Design review of the part built by this model. Coordinates are the model's own, in mm. Coordinates: 2 decimals unless noted, no trailing zeros. Write each loop counter-clockwise with the first axis right and the second up, starting at its lowest first coordinate (ties: lowest second). Pieces come first, ordered by that corner, then holes.
Q1. To check wall thickness, follow probe 1 along Y at (x, z) = (19, -5); probe 2 along Y at (x, z) = (-15, -7.25); probe 3 along X at (y, z) = (228.5, -3). State the ranges of each line that lie inside material, in increasing order.
Q2. Add section C-C, the plane y = 156. Give the boundary of the cut face in (x, z).
Q3. The part is to be moulded in two halves that separate along X. For faces 1 (the face through (-165, -153.2, -4.9)), 2 (the face through (-0.286, 264.503, -4.93)), 3 (the face through (165, 153.2, -4.9)), say which applies: +X half, -X half, draft (parallel to the pull), parting line (faces both ways), or undercut.
Q4. Add section A-A, the plane z = -6.75. Give the number of separate pieces and of enclosed holes in the cut face, plus the area to 3 significant figures.
Q5. Clearance check with flat-ended pins moving along their axes: pin 1 Ø2.5 at (x, y) = (-281.7, 8) entering from +Z; pin 2 Ø5 at (y, z) = (284, -4.5) entering from -X; pin 3 Ø5 at (x, z) = (41, -4) entering from +Y; pin 4 Ø1.5 at (y, z) = (-81, -1.5) entering from +X. State where each tip first meets the part, or that it passes through.
Q6. Add section B-B, the plane x = 0. Give the boundary of the cut face in (y, z), plus the area to 3 significant figures.
Autodesk Inventor part; units mm, degrees
ref_plane "YZ Plane" through (0, 0, 0) normal (1, 0, 0) x (0, 1, 0)
ref_plane "XZ Plane" through (0, 0, 0) normal (0, 1, 0) x (-1, 0, 0)
ref_plane "XY Plane" through (0, 0, 0) normal (0, 0, 1) x (1, 0, 0)
sketch "Sketch2" plane through (0, 0, 0) normal (0, 0, 1) x (1, 0, 0)
  circle A0 centre (0, 277.5) radius 8 construction
  circle A1 centre (0, 277.5) radius 13
  circle A2 centre (0, 277.5) radius 10.5 construction
  line L0 (25, 287.5) -> (-25, 287.5) construction
  line L1 (-25, 287.5) -> (-25, 222.5) construction
  line L2 (-25, 222.5) -> (25, 222.5) construction
  line L3 (25, 222.5) -> (25, 287.5) construction
  circle A3 centre (15, 228.5) radius 2.7
  circle A4 centre (-15, 228.5) radius 2.7
  circle A5 centre (-19, 277.5) radius 2.7
  circle A6 centre (19, 277.5) radius 2.7
  circle A7 centre (0, -277.5) radius 8 construction
  circle A8 centre (0, -277.5) radius 13
  circle A9 centre (0, -277.5) radius 10.5 construction
  line L4 (25, -287.5) -> (-25, -287.5) construction
  line L5 (-25, -287.5) -> (-25, -222.5) construction
  line L6 (-25, -222.5) -> (25, -222.5) construction
  line L7 (25, -222.5) -> (25, -287.5) construction
  circle A10 centre (-15, -228.5) radius 2.7
  circle A11 centre (15, -228.5) radius 2.7
  circle A12 centre (-19, -277.5) radius 2.7
  circle A13 centre (19, -277.5) radius 2.7
  line L8 (10.5, -277.5) -> (10.5, -287.5) construction
  line L9 (-10.5, -277.5) -> (-10.5, -287.5) construction
  line L10 (10.5, 277.5) -> (10.5, 287.5) construction
  line L11 (-10.5, 277.5) -> (-10.5, 287.5) construction
  circle A14 centre (281.7, 0) radius 5.25
  circle A15 centre (289.7, 0) radius 1.6
  circle A16 centre (281.7, 8) radius 1.6
  circle A17 centre (273.7, 0) radius 1.6
  circle A18 centre (281.7, -8) radius 1.6
  circle A19 centre (-281.7, 0) radius 5.25
  circle A20 centre (-289.7, 0) radius 1.6
  circle A21 centre (-281.7, -8) radius 1.6
  circle A22 centre (-273.7, 0) radius 1.6
  circle A23 centre (-281.7, 8) radius 1.6
  line L12 (0, -318.1981) -> (318.1981, 0)
  line L13 (318.1981, 0) -> (0, 318.1981)
  line L14 (0, 318.1981) -> (-318.1981, 0)
  line L15 (-318.1981, 0) -> (0, -318.1981)
  line L16 (0, -318.1981) -> (0, 318.1981) construction
  line L17 (318.1981, 0) -> (-318.1981, 0) construction
  line L18 (0, -318.1981) -> (450, -318.1981) construction
  line L19 (300.5, 17.6981) -> (300.5, -17.6981)
  line L20 (-300.5, 17.6981) -> (-300.5, -17.6981)
  line L21 (-20.6981, 297.5) -> (20.6981, 297.5) construction
  line L22 (-25.6981, 292.5) -> (25.6981, 292.5)
  line L23 (-20.6981, -297.5) -> (20.6981, -297.5) construction
  line L24 (-25.6981, -292.5) -> (25.6981, -292.5)
  line L25 (-9.5, 297.5) -> (-3.976, 284.442) construction
  line L26 (9.5, 297.5) -> (3.976, 284.442) construction
  line L27 (-14.929, 297.5) -> (-9.9883, 285.8207)
  line L28 (14.929, 297.5) -> (9.9883, 285.8207)
  line L29 (-9.5, -297.5) -> (-3.976, -284.442) construction
  line L30 (9.5, -297.5) -> (3.976, -284.442) construction
  line L31 (14.929, -297.5) -> (9.9883, -285.8207)
  line L32 (-14.929, -297.5) -> (-9.9883, -285.8207)
  line L33 (-13, 277.5) -> (-13, 292.5)
  line L34 (13, 277.5) -> (13, 292.5)
  line L35 (-13, -277.5) -> (-13, -292.5)
  line L36 (13, -277.5) -> (13, -292.5)
  line L37 (13, -277.5) -> (28, -277.5) construction
  point P0 (0, 0)
  point P1 (-12.8138, -292.5)
  point P2 (12.8138, -292.5)
  point P3 (12.8138, 292.5)
  point P4 (-12.8138, 292.5)
  point P5 (300.5, 292.5)
  point P6 (300.5, -292.5)
  point P7 (-300.5, -292.5)
  point P8 (-300.5, 292.5)
  dimension "d256" = 16
  dimension "d257" = 0
  dimension "d258" = 277.5
  dimension "d259" = 26
  dimension "d260" = 21
  dimension "d261" = 50
  dimension "d262" = 10
  dimension "d263" = 65
  dimension "d265" = 50
  dimension "d266" = 25
  dimension "d267" = 5.4
  dimension "d268" = 5.4
  dimension "d269" = 5.4
  dimension "d270" = 5.4
  dimension "d271" = 6
  dimension "d272" = 10
  dimension "d273" = 6
  dimension "d274" = 10
  dimension "d275" = 6
  dimension "d276" = 10
  dimension "d277" = 6
  dimension "d278" = 10
  dimension "d279" = 0
  dimension "d280" = 277.5
  dimension "d281" = 26
  dimension "d282" = 16
  dimension "d283" = 21
  dimension "d284" = 50
  dimension "d285" = 10
  dimension "d286" = 65
  dimension "d287" = 25
  dimension "d288" = 5.4
  dimension "d289" = 5.4
  dimension "d290" = 5.4
  dimension "d291" = 5.4
  dimension "d292" = 6
  dimension "d293" = 10
  dimension "d294" = 6
  dimension "d295" = 10
  dimension "d296" = 10
  dimension "d297" = 6
  dimension "d298" = 10
  dimension "d299" = 6
  dimension "d300" = 10.5
  dimension "d301" = 0
  dimension "d302" = 281.7
  dimension "d303" = 3.2
  dimension "d304" = 0
  dimension "d305" = 8
  dimension "d308" = 360
  dimension "d310" = 10.5
  dimension "d311" = 0
  dimension "d312" = 281.7
  dimension "d313" = 3.2
  dimension "d314" = 0
  dimension "d315" = 8
  dimension "d318" = 360
  dimension "d320" = 450
  dimension "d321" = 45
  dimension "d322" = 450
  dimension "d323" = 18.8
  dimension "d324" = 18.8
  dimension "d325" = 20
  dimension "d326" = 15
extrude "Extrusion11" add sketch "Sketch2" against normal blind 10 contours L34 L22 L13 L19 L12 L24 L36 A8 L35 L15 L20 L14 L33 A1
equation "\"dist_rails\" = 555"
equation "\"dist_leadscrews\" = 563.4"
equation "\"diam_leadscrew_hole\" = 10.5"
equation "\"delta\" = 5"
equation "\"rail_angle\" = 67.07deg"
equation "\"rail_D\" = 9.5"
equation "\"rail_diam\" = 16"
properties part number "z_plate" material "Aluminum 6061"
Here are the results:
1. probe 1: y = -292.5 to -280.2, -274.8 to 274.8, 280.2 to 292.5
1. probe 2: y = -292.5 to -231.2, -225.8 to 225.8, 231.2 to 292.5
1. probe 3: x = -89.7 to -17.7, -12.3 to 12.3, 17.7 to 89.7
2. outline: (-162.2, -10) - (162.2, -10) - (162.2, 0) - (-162.2, 0) - close
3. face 1: -X half
3. face 2: undercut
3. face 3: +X half
4. separate pieces: 1
4. enclosed holes: 18
4. area: 199,000 mm2
5. pin 1: passes through
5. pin 2: stops at x = -36.7
5. pin 3: stops at y = 279.7
5. pin 4: stops at x = 237.95
6. outline: (-264.5, -10) - (264.5, -10) - (264.5, 0) - (-264.5, 0) - close
6. area: 5,290 mm2
